Input: part model. Units: mm. Frame: model coordinates. Round coordinates to 2 decimals unless told otherwise and drop trailing zeros. Loops run counter-clockwise (first coordinate to the right, second up) from the corner with the lowest first, then second, coordinate; pieces in that order, holes last.
(1) Line query: line 1 (X direction, y = 0, z = 2.8); line 2 (X direction, y = -0.4, z = 4.35). Output: solid intervals per line, ascending.
(2) Draft query along Y for faces 1 (the face through (0.323, 0.506, 2.218)), 2 (the face through (3, 0, 2)), 3 (the face through (0, -3, 2)), 4 (the face through (0, 3, 2)). Return one class per face: released by +Y, released by -Y, zero draft, split by the parting line, or undercut.
(3) Cut plane A-A, the plane y = 0. Output: boundary loops of the cut face in (x, z).
(4) Cut plane C-C, the plane z = 2.95. Output: boundary loops of the cut face in (x, y).
from build123d import *

# Parameters (mm, degrees)
CYLINDER_R     = 0.6
CYLINDER_DEPTH = 10
BOX008_W       = 6
BOX008_H       = 6
BOX008_DEPTH   = 4.5


with BuildPart() as hole:
    # Cylinder → Cylinder (new body)
    with BuildSketch(Plane.XY):
        Circle(CYLINDER_R)
    extrude(amount=CYLINDER_DEPTH)


with BuildPart() as stand_hole_cut:
    # Box008 → Box008 (new body)
    with BuildSketch(Plane(origin=(-3, -3, 0), x_dir=(1, 0, 0), z_dir=(0, 0, 1))):
        with Locations((3, 3)):
            Rectangle(BOX008_W, BOX008_H)
    extrude(amount=BOX008_DEPTH)

    # Cut003002: cut hole
    add(hole.part, mode=Mode.SUBTRACT)


solid = stand_hole_cut.part
Reported:
1. line 1: x = -3 to -0.6, 0.6 to 3
1. line 2: x = -3 to -0.45, 0.45 to 3
2. face 1: undercut
2. face 2: zero draft
2. face 3: released by -Y
2. face 4: released by +Y
3. outline: (-3, 0) - (-0.6, 0) - (-0.6, 4.5) - (-3, 4.5) - close; (0.6, 0) - (3, 0) - (3, 4.5) - (0.6, 4.5) - close
4. outline: (-3, -3) - (3, -3) - (3, 3) - (-3, 3) - close; hole circle Ø1.2 at (0, 0)
